The figure shows three views and two pictorial views of one solid part (mm, origin at its lowest corner). Answer the questions. A direction names the side the tool comes from. Coordinates: 2 decimals unless noted, no trailing zeros. Write each loop counter-clockwise with the first axis right and the second up, starting at its lowest first coordinate (ties: lowest second). Pieces come first, ordered by that corner, then holes.
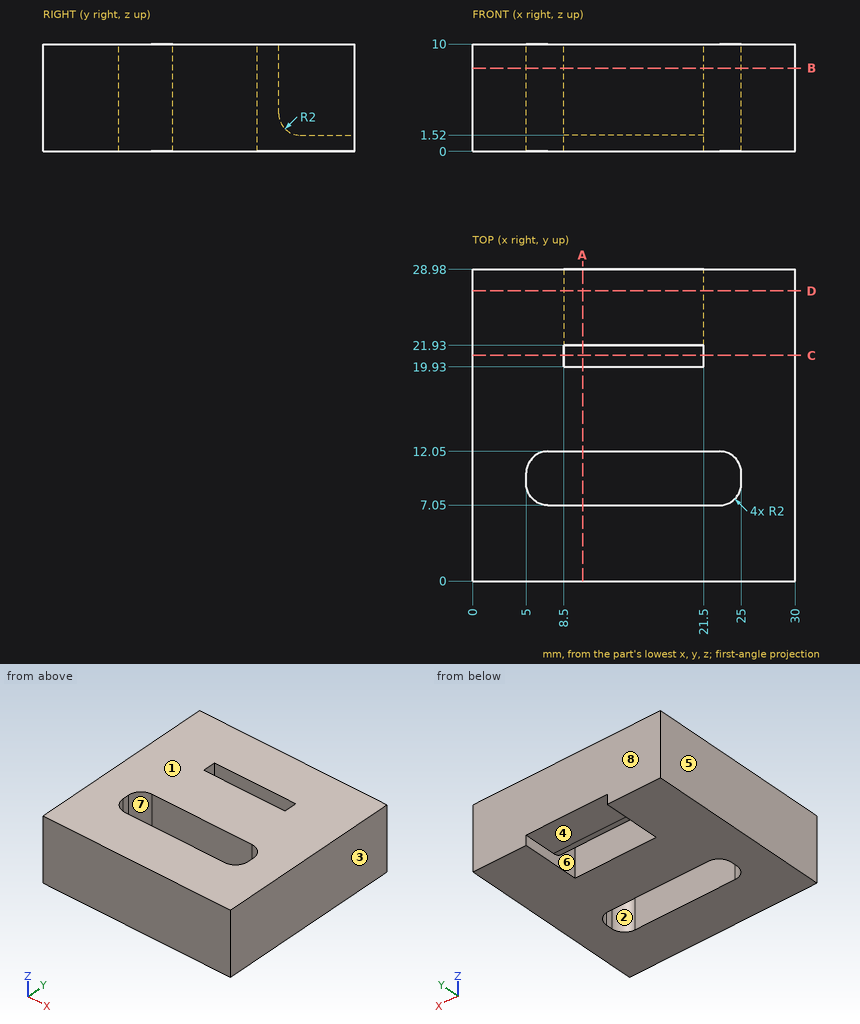
1. Section C-C on y = 21 is taken. Give the vertices of the cut face in (x, z).
Results found:
outline: (0, 0) - (8.5, 0) - (8.5, 10) - (0, 10) - close; (21.5, 0) - (30, 0) - (30, 10) - (21.5, 10) - close
2. A tool of negligible diameter and unlimited length cuts with its end or side. For the marked faces 4, 5, 6, 7 and 8, from which of +Z, -Z, +X, -X, +Y, -Y can it reach the whole face along a straight path? Write none if from no direction.
Results found:
face 4: -Z, +Y
face 5: +Z, -Z, -X, +Y, -Y
face 6: -Z
face 7: +Z, -Z
face 8: +Z, -Z, +X, -X, +Y
3. Section A-A on x = 10.25 is taken. Give the vertices of the cut face in (y, z).
Results found:
outline: (0, 0) - (7.05, 0) - (7.05, 10) - (0, 10) - close; (12.05, 0) - (19.93, 0) - (19.93, 10) - (12.05, 10) - close; (21.93, 3.52) arc R2 ccw to (23.93, 1.52) - (28.98, 1.52) - (28.98, 10) - (21.93, 10) - close
4. A flat-ended cylindrical pin translates along its axis: P1, Ø5.5, axis at x = 15, y = 25.5, coming from the -Z side. Find the tip coordinate at first contact, or state that the pin passes through.
Results found:
P1: stops at z = 1.52
5. For a pull along X with two mould halves and no side action, classify the marked faces 1, 2 and 3 as pulls with the +X half, pulls with the -X half, needs draft (parallel to the pull), parting line crosses it, or undercut.
Results found:
face 1: needs draft
face 2: undercut
face 3: pulls with the +X half
6. Section D-D on y = 27 is taken. Give the vertices of the cut face in (x, z), then the cut area to 3 significant figures.
Results found:
outline: (0, 0) - (8.5, 0) - (8.5, 1.52) - (21.5, 1.52) - (21.5, 0) - (30, 0) - (30, 10) - (0, 10) - close
area: 280 mm2
7. Section B-B on z = 7.75 is taken. Give the vertices of the cut face in (x, y), then the cut area to 3 significant figures.
Results found:
outline: (0, 0) - (30, 0) - (30, 28.98) - (0, 28.98) - close; hole (5, 9.05) arc R2 ccw to (7, 7.05) - (23, 7.05) arc R2 ccw to (25, 9.05) - (25, 10.05) arc R2 ccw to (23, 12.05) - (7, 12.05) arc R2 ccw to (5, 10.05) - close; hole (8.5, 19.93) - (21.5, 19.93) - (21.5, 21.93) - (8.5, 21.93) - close
area: 747 mm2
8. Find the intervals of material crossed by L1, parallel to Y at x = 10.75, z = 8.25; L2, parallel to X at y = 20.75, z = 9.75; L3, parallel to X at y = 10, z = 8.5, in increasing order.
Results found:
L1: y = 0 to 7.05, 12.05 to 19.93, 21.93 to 28.98
L2: x = 0 to 8.5, 21.5 to 30
L3: x = 0 to 5, 25 to 30
